The figure shows three views and two pictorial views of one solid part (mm, origin at its lowest corner). Answer the questions. A direction names the side the tool comes from. Coordinates: 2 decimals unless noted, no trailing zeros. Write each loop counter-clockwise with the first axis right and the second up, starting at its lowest first coordinate (ties: lowest second). Pieces come first, ordered by that corner, then holes. Notation, with made-up numbers: M -29,-20.75 L 21,-20.75 A11 ccw 21,-7.75 Z; hole C 72,17.25 d11. An arc over 180 degrees is marked long. Use CSV: the item, a comma, the result in double quotes.
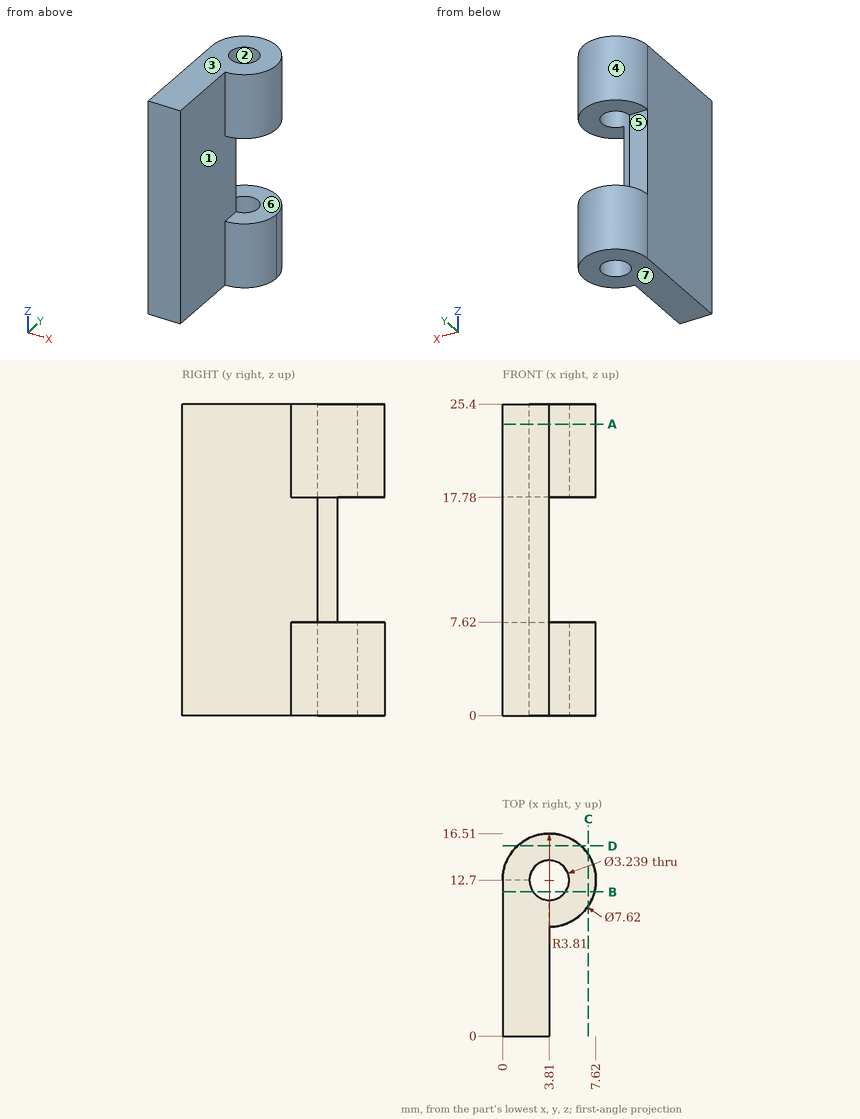
Item 1: The part is cut by section A-A (z = 23.75). Write down the section's boundary in (x, y).
Answer:
outline,"M 0,0 L 3.81,0 L 3.81,8.89 A3.81 ccw long 0,12.7 Z; hole C 3.81,12.7 d3.24"
Item 2: For a pull along X with two mould halves and no side action, classify the marked faces 1, 2, 3 and 4 as released by +X, released by -X, zero draft, split by the parting line, or undercut.
Answer:
face 1,"released by +X"
face 2,"undercut"
face 3,"zero draft"
face 4,"split by the parting line"
Item 3: Given pin 1 (5 mm diameter, centred on y = 12.5, z = 12, fed in from +X); pin 2 (3 mm diameter, centred on x = 6, y = 7, fed in from -Z); pin 3 (1.8 mm diameter, centred on x = 1, z = 12, fed in from +Y), each flat-ended and moving along its own axis, determine where each tip first touches the part or whether it passes through.
Answer:
pin 1,"stops at x = 3.81"
pin 2,"passes through"
pin 3,"stops at y = 12.7"
Item 4: The part is cut by section C-C (x = 7). Write down the section's boundary in (y, z).
Answer:
outline,"M 10.62,0 L 14.78,0 L 14.78,7.62 L 10.62,7.62 Z; M 10.62,17.78 L 14.78,17.78 L 14.78,25.4 L 10.62,25.4 Z"
Item 5: The part is cut by section B-B (y = 11.75). Write down the section's boundary in (x, z).
Answer:
outline,"M 0,0 L 2.5,0 L 2.5,25.4 L 0,25.4 Z; M 5.12,0 L 7.5,0 L 7.5,7.62 L 5.12,7.62 Z; M 5.12,17.78 L 7.5,17.78 L 7.5,25.4 L 5.12,25.4 Z"
Item 6: A tool of negligible diameter and unlimited length cuts with its end or side. For the marked faces 5, 6 and 7, from which of +Z, -Z, +X, -X, +Y, -Y can it reach the whole face along a straight path? Write none if from no direction.
Answer:
face 5,"+X, -X, +Y"
face 6,"+X, +Y"
face 7,"-Z, +X, -X, +Y, -Y"
Item 7: The part is cut by section D-D (y = 15.5). Write down the section's boundary in (x, z).
Answer:
outline,"M 1.23,0 L 6.39,0 L 6.39,7.62 L 1.23,7.62 Z; M 1.23,17.78 L 6.39,17.78 L 6.39,25.4 L 1.23,25.4 Z"
Item 8: Consider probe 1 along Z at (x, y) = (6.25, 10.25); probe 2 along Y at (x, z) = (1, 16.25); probe 3 along X at (y, z) = (6.75, 14.25). Determine where each line is inside the solid, lowest interval first.
Answer:
probe 1,"z = 0 to 7.62, 17.78 to 25.4"
probe 2,"y = 0 to 12.7"
probe 3,"x = 0 to 3.81"
